Work out the finished part from the listing and answer in its coordinate system (mm). A direction names the side the tool comes from. Round coordinates to 2 decimals unless told otherwise and drop trailing zeros. Order: outer loops, then holes, each group sorted by start corner. A loop starts at its lowest first (then second) coordinate and runs counter-clockwise, first axis right, second up. Notation, with made-up numbers: (31, 58) - (61, 58) arc R20 ccw to (61, 78) - close; hole circle Ø9 at (6, 19.25). An arc over 180 degrees is marked (long way). Put each result on its own line as item: value.
```python
from build123d import *

# Parameters (mm, degrees)
SKETCH1_W           = 139.7
SKETCH1_H           = 66.04
BOSS_EXTRUDE1_DEPTH = 13.208
SKETCH2_W           = 38.1
SKETCH2_H           = 53.34
CUT_EXTRUDE1_DEPTH  = 13.208
SKETCH3_W           = 38.1
SKETCH3_H           = 12.7
BOSS_EXTRUDE2_DEPTH = 31.242
SKETCH4_W           = 12.7
SKETCH4_H           = 23.368
CUT_EXTRUDE2_DEPTH  = 3.556
SKETCH5_W           = 17.018
SKETCH5_H           = 22.606
SKETCH5_W_2         = 4.318
SKETCH5_H_2         = 10.414
BOSS_EXTRUDE3_DEPTH = 9.525
SKETCH6_W           = 7.366
SKETCH6_H           = 7.366
SKETCH6_W_2         = 13.208
SKETCH6_H_2         = 8.128
CUT_EXTRUDE3_DEPTH  = 172.847
BOSS_EXTRUDE4_DEPTH = 139.7
SKETCH8_W           = 133.35
SKETCH8_H           = 12.7
CUT_EXTRUDE4_DEPTH  = 139.7
SKETCH9_W           = 38.1
SKETCH9_H           = 31.496
CUT_EXTRUDE5_DEPTH  = 139.7
SKETCH10_W          = 38.1
SKETCH10_H          = 8.382
CUT_EXTRUDE6_DEPTH  = 139.7


with BuildPart() as part:
    # Sketch1 → Boss-Extrude1 (new body)
    with BuildSketch(Plane.XY):
        with Locations((69.85, 33.02)):
            Rectangle(SKETCH1_W, SKETCH1_H)
    extrude(amount=BOSS_EXTRUDE1_DEPTH)

    # Sketch2 → Cut-Extrude1 (cut)
    with BuildSketch(Plane.XY.offset(13.208)):
        with Locations((69.85, 39.37)):
            Rectangle(SKETCH2_W, SKETCH2_H)
    extrude(amount=-CUT_EXTRUDE1_DEPTH, mode=Mode.SUBTRACT)

    # Sketch3 → Boss-Extrude2 (add)
    with BuildSketch(Plane.XY.offset(13.208)):
        with Locations((69.85, 6.35)):
            Rectangle(SKETCH3_W, SKETCH3_H)
    extrude(amount=BOSS_EXTRUDE2_DEPTH)

    # Sketch4 → Cut-Extrude2 (cut)
    with BuildSketch(Plane(origin=(0, 12.7, 0), x_dir=(1, 0, 0), z_dir=(0, 1, 0))):
        with Locations((69.85, -18.034)):
            Rectangle(SKETCH4_W, SKETCH4_H)
    extrude(amount=-CUT_EXTRUDE2_DEPTH, mode=Mode.SUBTRACT)

    # Sketch5 → Boss-Extrude3 (add)
    with BuildSketch(Plane.XZ):
        with Locations((69.85, 11.303)):
            Rectangle(SKETCH5_W, SKETCH5_H)
        with Locations((69.85, 11.557)):
            Rectangle(SKETCH5_W_2, SKETCH5_H_2, mode=Mode.SUBTRACT)
    extrude(amount=BOSS_EXTRUDE3_DEPTH)

    # Sketch6 → Cut-Extrude3 (cut)
    with BuildSketch(Plane(origin=(139.7, 0, 0), x_dir=(0, 0, -1), z_dir=(1, 0, 0))):
        with Locations((-3.683, 47.879)):
            Rectangle(SKETCH6_W, SKETCH6_H)
        with Locations((-6.604, 61.976)):
            Rectangle(SKETCH6_W_2, SKETCH6_H_2)
    extrude(amount=-CUT_EXTRUDE3_DEPTH, mode=Mode.SUBTRACT)

    # Sketch7 → Boss-Extrude4 (add)
    with BuildSketch(Plane.ZY):
        Polygon((0, 59.944), (0, 70.612), (13.208, 70.612), (13.208, 59.944), (13.208, 57.912), (10.033, 57.912), (10.033, 59.944), (10.033, 67.437), (3.175, 67.437), (3.175, 59.944), align=None)
    extrude(amount=-BOSS_EXTRUDE4_DEPTH)

    # Sketch8 → Cut-Extrude4 (cut)
    with BuildSketch(Plane.XY.offset(13.208)):
        with Locations((69.85, 64.262)):
            Rectangle(SKETCH8_W, SKETCH8_H)
    extrude(amount=-CUT_EXTRUDE4_DEPTH, mode=Mode.SUBTRACT)

    # Sketch9 → Cut-Extrude5 (cut)
    with BuildSketch(Plane(origin=(0, 0, 0), x_dir=(-1, 0, 0), z_dir=(0, 0, -1))):
        with Locations((-120.65, 15.748)):
            Rectangle(SKETCH9_W, SKETCH9_H)
        with Locations((-19.05, 15.748)):
            Rectangle(SKETCH9_W, SKETCH9_H)
    extrude(amount=-CUT_EXTRUDE5_DEPTH, mode=Mode.SUBTRACT)

    # Sketch10 → Cut-Extrude6 (cut)
    with BuildSketch(Plane(origin=(0, 12.7, 0), x_dir=(1, 0, 0), z_dir=(0, 1, 0))):
        with Locations((69.85, -40.259)):
            Rectangle(SKETCH10_W, SKETCH10_H)
    extrude(amount=-CUT_EXTRUDE6_DEPTH, mode=Mode.SUBTRACT)


solid = part.part
```
1) For faces 4 (the flat face through (70, -5, 16.764)), 5 (the flat face through (50.8, 6, 24)), 6 (the flat face through (138, 63, 10.033)), determine the directions among +Z, -Z, +X, -X, +Y, -Y from which every point of the face is accessible in a straight line to the end or side of a thin tool.
Findings below:
face 4: -Y
face 5: +Z, -X, +Y, -Y
face 6: +X, -X
2) Given pin 1 Ø1.6 at (x, z) = (138, 7.5) entering from -Y; pin 2 Ø14.5 at (y, z) = (17, 6) entering from +X; pin 3 Ø5 at (x, z) = (65.5, 22.5) entering from +Y, each flat-ended and moving along its own axis, determine where each tip first touches the part or whether it passes through.
Findings below:
pin 1: stops at y = 31.5
pin 2: stops at x = 101.6
pin 3: stops at y = 12.7
3) A cutting plane is placed at C-C on x = 9. Write down the section's boundary in (y, z), then the cut area to 3 significant figures.
Findings below:
outline: (31.5, 0) - (44.2, 0) - (44.2, 7.37) - (51.56, 7.37) - (51.56, 0) - (57.91, 0) - (57.91, 13.21) - (31.5, 13.21) - close
area: 295 mm2
4) A cutting plane is placed at B-B on y = 47.5. Write down the section's boundary in (x, z), then the cut area to 3 significant figures.
Findings below:
outline: (0, 7.37) - (50.8, 7.37) - (50.8, 13.21) - (0, 13.21) - close; (88.9, 7.37) - (139.7, 7.37) - (139.7, 13.21) - (88.9, 13.21) - close
area: 594 mm2
5) A cutting plane is placed at D-D on z = 19. Write down the section's boundary in (x, y) (3 decimals).
Findings below:
outline: (50.8, 0) - (61.341, 0) - (61.341, -9.525) - (78.359, -9.525) - (78.359, 0) - (88.9, 0) - (88.9, 12.7) - (76.2, 12.7) - (76.2, 9.144) - (63.5, 9.144) - (63.5, 12.7) - (50.8, 12.7) - close
6) A cutting plane is placed at A-A on y = 63. Write down the section's boundary in (x, z) (3 decimals).
Findings below:
outline: (0, 0) - (3.175, 0) - (3.175, 3.175) - (0, 3.175) - close; (0, 10.033) - (3.175, 10.033) - (3.175, 13.208) - (0, 13.208) - close; (136.525, 0) - (139.7, 0) - (139.7, 3.175) - (136.525, 3.175) - close; (136.525, 10.033) - (139.7, 10.033) - (139.7, 13.208) - (136.525, 13.208) - close
7) Straight lines are drawn through the part: L1, parallel to X at y = 66.5, z = 10.5 (3 decimals); L2, parallel to X at y = 9.5, z = 18.5; L3, parallel to Y at x = 64, z = 15 (3 decimals). For each, find the intervals that lie inside material, in ascending order. Write a range as from..to.
Findings below:
L1: x = 0..3.175, 136.525..139.7
L2: x = 50.8..63.5, 76.2..88.9
L3: y = -9.525..9.144
8) For a pull along Z with two mould halves and no side action, classify faces 1 (the flat face through (138, 67.437, 7)), 2 (the flat face through (88.9, 35, 7)), 3 (the flat face through (26, 48, 7.366)) as pulls with the +Z half, pulls with the -Z half, needs draft (parallel to the pull), parting line crosses it, or undercut.
Findings below:
face 1: undercut
face 2: needs draft
face 3: pulls with the -Z half
